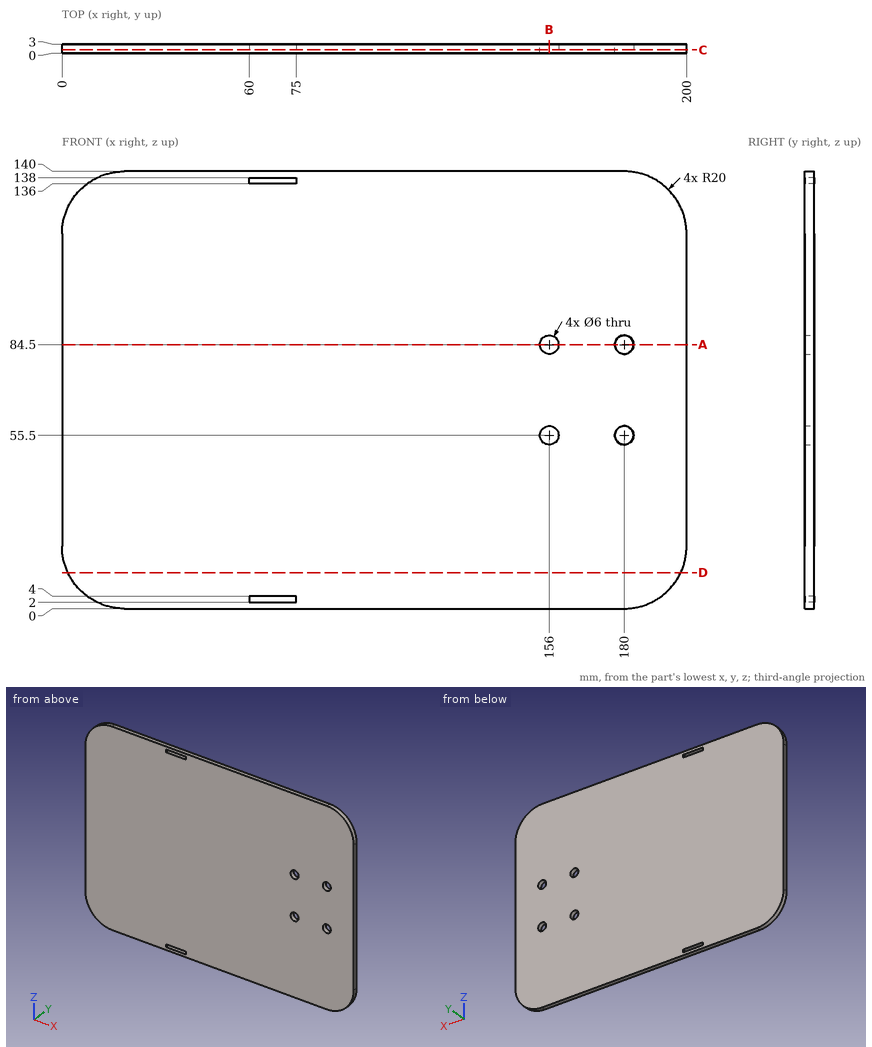
Check sheet for the drawn part. Datum: minimum x, y, z corner. Units: mm. Coordinates: 2 decimals unless noted, no trailing zeros. Loops run counter-clockwise (first coordinate to the right, second up) from the corner with the lowest first, then second, coordinate; pieces in that order, holes last. Notation, with made-up numbers: (66, 79.5) -> (88, 79.5) arc R8 cw to (88, 92.5) -> close; hole circle Ø3 at (1, 47.25). An arc over 180 degrees is marked (long way). Answer in a Markdown table with one row per item.
1) Section check A-A (z = 84.5). Record the cut outline in (x, y), and give its area (3 significant figures).
The answers:
| item | result |
|---|---|
| outline | (0, 0) -> (153, 0) -> (153, 3) -> (0, 3) -> close; (159, 0) -> (177, 0) -> (177, 3) -> (159, 3) -> close; (183, 0) -> (200, 0) -> (200, 3) -> (183, 3) -> close |
| area | 564 mm2 |
2) Scan lines: line 1 along Z through (x, y) = (180, 0.85); line 2 along X through (y, z) = (1.05, 55.5); line 3 along Z through (x, y) = (64.5, 2.4). Record each from-to range of solid material in increasing order. Write a range as from..to.
The answers:
| item | result |
|---|---|
| line 1 | z = 0..52.5, 58.5..81.5, 87.5..140 |
| line 2 | x = 0..153, 159..177, 183..200 |
| line 3 | z = 0..2, 4..136, 138..140 |
3) Section check B-B (x = 156). Record the cut outline in (y, z).
The answers:
| item | result |
|---|---|
| outline | (0, 0) -> (3, 0) -> (3, 52.5) -> (0, 52.5) -> close; (0, 58.5) -> (3, 58.5) -> (3, 81.5) -> (0, 81.5) -> close; (0, 87.5) -> (3, 87.5) -> (3, 140) -> (0, 140) -> close |
4) Section check C-C (y = 1.15). Record the cut outline in (x, z), and give its area (3 significant figures).
The answers:
| item | result |
|---|---|
| outline | (0, 20) arc R20 ccw to (20, 0) -> (180, 0) arc R20 ccw to (200, 20) -> (200, 120) arc R20 ccw to (180, 140) -> (20, 140) arc R20 ccw to (0, 120) -> close; hole (60, 2) -> (75, 2) -> (75, 4) -> (60, 4) -> close; hole (60, 136) -> (75, 136) -> (75, 138) -> (60, 138) -> close; hole circle Ø6 at (156, 55.5); hole circle Ø6 at (156, 84.5); hole circle Ø6 at (180, 55.5); hole circle Ø6 at (180, 84.5) |
| area | 27,500 mm2 |
5) Depth check by flat-ended pin: P1, Ø1.6, axis at y = 2, z = 3, coming from the -X side. Enter the tip coordinate at first touch or a pass-through.
The answers:
| item | result |
|---|---|
| P1 | stops at x = 8.27 |
6) Section check D-D (z = 11.5). Record the cut outline in (x, y), and give its area (3 significant figures).
The answers:
| item | result |
|---|---|
| outline | (1.9, 0) -> (198.1, 0) -> (198.1, 3) -> (1.9, 3) -> close |
| area | 589 mm2 |
